from build123d import *

# Parameters (mm, degrees)
SKETCH1_R           = 22.86
BOSS_EXTRUDE1_DEPTH = 12.7
SKETCH2_R           = 22.225
CUT_EXTRUDE1_DEPTH  = 10.16
SKETCH3_R           = 12.7
BOSS_EXTRUDE2_DEPTH = 15.24


with BuildPart() as part:
    # Sketch1 → Boss-Extrude1 (new body)
    with BuildSketch(Plane.XY):
        Circle(SKETCH1_R)
    extrude(amount=BOSS_EXTRUDE1_DEPTH)

    # Sketch2 → Cut-Extrude1 (cut)
    with BuildSketch(Plane.XY.offset(12.7)):
        Circle(SKETCH2_R)
    extrude(amount=-CUT_EXTRUDE1_DEPTH, mode=Mode.SUBTRACT)

    # Sketch3 → Boss-Extrude2 (add)
    with BuildSketch(Plane.XY.offset(2.54)):
        with Locations(Location((0, 0, 0), (0, 0, 180))):
            Circle(SKETCH3_R)
    extrude(amount=BOSS_EXTRUDE2_DEPTH)


solid = part.part
Design review of the part built by this model. Coordinates are the model's own, in mm. A direction names the side the tool comes from. Give positions to 0.01 mm unless a question says otherwise; leave off trailing zeros. Order: outer loops, then holes, each group sorted by start corner. A loop starts at its lowest first (then second) coordinate and runs counter-clockwise, first axis right, second up. Notation, with made-up numbers: (12.25, -24) - (60.25, -24) arc R27 cw to (60.25, 15) - close; hole circle Ø8 at (-1.75, 8). An arc over 180 degrees is marked (long way). Write item = value, one per line. Start each with the question number.
Q1. We need section A-A on y = 0. State the section outline as (x, z) points (3 decimals).
Q2. Mouldability with a two-part tool opening along X and no side actions: class faces 1 (the face through (0, 0, 0)), 2 (the face through (21.199, 6.676, 7.691)), 3 (the face through (21.804, 6.867, 6.261)) as released by +X, released by -X, zero draft, split by the parting line, or undercut.
Q3. To check wall thickness, follow L1, parallel to Y at x = 0, z = 10.25 (3 decimals); L2, parallel to Y at x = -2, z = 2.75; L3, parallel to Z at x = -16.5, y = 15. State the ranges of each line that lie inside material, in increasing order. Write a range as from..to.
Q4. We need section B-B on z = 11.25. State the section outline as (x, y) points (3 decimals).
Q5. Clearance check with flat-ended pins moving along their axes: pin 1 Ø5 at (x, y) = (14.5, -14.5) entering from +Z; pin 2 Ø5 at (y, z) = (8.5, 7) entering from +X; pin 3 Ø2 at (x, z) = (12, 14.5) entering from +Y. State where each tip first meets the part, or that it passes through.
Q6. We need section D-D on z = 1. State the section outline as (x, y) points.
Q7. Tool access review of faces 4 (the face through (0, 0, 17.78)), 5 (the face through (10, -10, 2.54)): name each direction out of +Z, -Z, +X, -X, +Y, -Y from which nothing blocks a thin tool from reaching the whole face with its end or side.
Working result:
q1.outline = (-22.86, 0) - (22.86, 0) - (22.86, 12.7) - (22.225, 12.7) - (22.225, 2.54) - (12.7, 2.54) - (12.7, 17.78) - (-12.7, 17.78) - (-12.7, 2.54) - (-22.225, 2.54) - (-22.225, 12.7) - (-22.86, 12.7) - close
q2.face_1 = zero draft
q2.face_2 = undercut
q2.face_3 = split by the parting line
q3.L1 = -22.86..-22.225, -12.7..12.7, 22.225..22.86
q3.L2 = -22.77..-22.13, -12.54..12.54, 22.13..22.77
q3.L3 = 0..12.7
q4.outline = circle Ø45.72 at (0, 0); circle Ø25.4 at (0, 0); hole circle Ø44.45 at (0, 0)
q5.pin_1 = 12.7
q5.pin_2 = 22.06
q5.pin_3 = 6.35
q6.outline = circle Ø45.72 at (0, 0)
q7.face_4 = +Z, +X, -X, +Y, -Y
q7.face_5 = +Z
